```python
from build123d import *

# Parameters (mm, degrees)
ESBO_O1_R                = 11
RESSALTO_EXTRUS_O1_DEPTH = 62
CORTE_EXTRUS_O1_START    = -14
ESBO_O2_R                = 11
CORTE_EXTRUS_O1_DEPTH    = 14


with BuildPart() as part:
    # Esboço1 → Ressalto-extrusão1 (new body)
    with BuildSketch(Plane.YZ):
        with Locations(Location((0, 0, 0), (0, 0, 270))):
            Circle(ESBO_O1_R)
    extrude(amount=RESSALTO_EXTRUS_O1_DEPTH)

    # Esboço2 → Corte-extrusão1 (cut)
    with BuildSketch(Plane.YZ.offset(62).offset(CORTE_EXTRUS_O1_START)):
        with Locations(Location((0, 0, 0), (0, 0, 270))):
            Circle(ESBO_O2_R)
        Polygon((0, 7.505553499), (-6.5, 3.75277675), (-6.5, -3.75277675), (0, -7.505553499), (6.5, -3.75277675), (6.5, 3.75277675), align=None, mode=Mode.SUBTRACT)
    extrude(amount=CORTE_EXTRUS_O1_DEPTH, mode=Mode.SUBTRACT)


solid = part.part
```
Design review of the part built by this model. Coordinates are the model's own, in mm. A direction names the side the tool comes from. Coordinates: 2 decimals unless noted, no trailing zeros. Order: outer loops, then holes, each group sorted by start corner. A loop starts at its lowest first (then second) coordinate and runs counter-clockwise, first axis right, second up. Notation, with made-up numbers: (41.5, 2.5) - (59.5, 2.5) arc R18 ccw to (59.5, 30.5) - close; hole circle Ø11 at (20, 8). An arc over 180 degrees is marked (long way). Answer in a Markdown table with one row per item.
(1) Clearance check with flat-ended pins moving along their axes: pin 1 (2 mm diameter, centred on x = 10.5, y = -7.5, fed in from +Z); pin 2 (4 mm diameter, centred on x = 14, z = 4.5, fed in from +Y); pin 3 (8.5 mm diameter, centred on x = 55.5, z = -0.5, fed in from +Y). State where each tip first meets the part, or that it passes through.
Checked values:
| item | result |
|---|---|
| pin 1 | z = 8.87 |
| pin 2 | y = 10.71 |
| pin 3 | y = 6.5 |
(2) Consider section B-B on y = 3.25. State the section outline as (x, z) points, plus the area to 3 significant figures.
Checked values:
| item | result |
|---|---|
| outline | (0, -10.51) - (48, -10.51) - (48, -5.63) - (62, -5.63) - (62, 5.63) - (48, 5.63) - (48, 10.51) - (0, 10.51) - close |
| area | 1,170 mm^2 |
(3) For faces 1 (the flat face through (54.9, -3.3, -5.6)), 2 (the flat face through (55, -6.5, 0)), 3 (the flat face through (54.9, 3.2, -5.66)), list the 3-axis set-ups (+Z, -Z, +X, -X, +Y, -Y) from which the entire face can be reached by the end or side of a thin tool; tool diameter is ignored.
Checked values:
| item | result |
|---|---|
| face 1 | -Z, +X, -Y |
| face 2 | +Z, -Z, +X, -Y |
| face 3 | -Z, +X, +Y |
(4) Consider section A-A on z = 0. State the section outline as (x, y) points, plus the area to 3 significant figures.
Checked values:
| item | result |
|---|---|
| outline | (0, -11) - (48, -11) - (48, -6.5) - (62, -6.5) - (62, 6.5) - (48, 6.5) - (48, 11) - (0, 11) - close |
| area | 1,240 mm^2 |
(5) Consider section D-D on y = -8.25. State the section outline as (x, z) points.
Checked values:
| item | result |
|---|---|
| outline | (0, -7.28) - (48, -7.28) - (48, 7.28) - (0, 7.28) - close |
(6) Consider section C-C on x = 29.5. State the section outline as (y, z) points.
Checked values:
| item | result |
|---|---|
| outline | circle Ø22 at (0, 0) |
(7) Wall thickness on line 1 along X through (y, z) = (-6.25, 8); line 2 along Z through (x, y) = (13, 0.5); line 3 along Y through (x, z) = (53.5, -1): over which ranges is each line inside the solid? List them lowest first. Write a range as from..to.
Checked values:
| item | result |
|---|---|
| line 1 | 0..48 |
| line 2 | -10.99..10.99 |
| line 3 | -6.5..6.5 |
